Geometry check sheet. Reference: the model listing, model coordinates, mm. A direction names the side the tool comes from. Give positions to 0.01 mm unless a question says otherwise; leave off trailing zeros. Loops run counter-clockwise (first coordinate to the right, second up) from the corner with the lowest first, then second, coordinate; pieces in that order, holes last. Notation, with made-up numbers: (10.25, 52) - (55.25, 52) arc R15 cw to (55.25, 65) - close; hole circle Ø9 at (89, 78.25). An arc over 180 degrees is marked (long way). Use a Markdown table: item, result. Add a question column.
1. Depth check by flat-ended pin: P1, Ø2, axis at x = 217.5, y = -21.5, coming from the +Z side; P2, Ø1.5, axis at x = 241.5, z = -337, coming from the -Y side. Enter the tip coordinate at first touch or a pass-through.
2. Cross-section at B-B on z = -172. Enter the section's corners in (x, y), and give its area (3 significant figures).
3. Material ranges on L1, parallel to Z at x = 308.5, y = -4.5; L2, parallel to X at y = -22.75, z = -360; L3, parallel to Y at x = 265, z = -382.5, recorded low to high.
4. Draft check along Z on faces 3 (the cylindrical face through (7.765, -12.522, -456.036)), 4 (the cylindrical face through (354.185, -12.522, -7.514)), 5 (the flat face through (179, -11, 0)), 6 (the cylindrical face through (356.52, -11.11, -457.82)). Enter one of: pulls with the +Z half, pulls with the -Z half, needs draft (parallel to the pull), parting line crosses it, or undercut.
5. Cross-section at A-A on y = -19.5. Enter the section's corners in (x, z), and give its area (3 significant figures).
6. Set-up check for faces 1 (the cylindrical face through (7.514, -12.522, -7.765)), 2 (the flat face through (0, -11, -235)): record each of +Z, -Z, +X, -X, +Y, -Y from which the full face is reachable in a straight line by a thin tool's end or side.
7. Cross-section at C-C on x = 133. Enter the section's corners in (y, z), and give its area (3 significant figures).
Autodesk Inventor part; units mm, degrees
ref_plane "YZ Plane" through (0, 0, 0) normal (1, 0, 0) x (0, 1, 0)
ref_plane "XZ Plane" through (0, 0, 0) normal (0, 1, 0) x (-1, 0, 0)
ref_plane "XY Plane" through (0, 0, 0) normal (0, 0, 1) x (1, 0, 0)
sketch "Sketch1" plane through (0, 0, 0) normal (0, 1, 0) x (-1, 0, 0)
  line L0 (0, 0) -> (-361.95, 0)
  line L1 (-361.95, 0) -> (-361.95, -463.55)
  line L2 (-361.95, -463.55) -> (0, -463.55)
  line L3 (0, -463.55) -> (0, 0)
  dimension "d0" = 361.95
  dimension "d1" = 463.55
extrude "Extrusion1" add sketch "Sketch1" along normal blind 2.794
fillet "Fillet1" radius 19.05 4 edges at (361.95, 1.397, 0) (361.95, 1.397, -463.55) (0, 1.397, -463.55) (0, 1.397, 0)
sketch "Sketch4" plane through (0, 0, 0) normal (0, -1, 0) x (1, 0, 0)
  point P0 (0, 0)
sketch "Sketch5" plane through (0, 0, 0) normal (0, -1, 0) x (1, 0, 0)
  arc A0 (19.05, 0) -> (0, -19.05) centre (19.05, -19.05) ccw
  line L0 (19.05, 0) -> (342.9, 0)
  line L1 (0, -444.5) -> (0, -19.05)
  line L2 (361.95, -19.05) -> (361.95, -444.5)
  arc A1 (361.95, -19.05) -> (342.9, 0) centre (342.9, -19.05) ccw
  arc A2 (0, -444.5) -> (19.05, -463.55) centre (19.05, -444.5) ccw
  line L3 (342.9, -463.55) -> (19.05, -463.55)
  arc A3 (342.9, -463.55) -> (361.95, -444.5) centre (342.9, -444.5) ccw
  arc A4 (2.9117, -444.5) -> (19.05, -460.6383) centre (19.05, -444.5) ccw
  line L4 (2.9117, -444.5) -> (2.9117, -19.05)
  arc A5 (19.05, -2.9117) -> (2.9117, -19.05) centre (19.05, -19.05) ccw
  line L5 (19.05, -2.9117) -> (342.9, -2.9117)
  arc A6 (359.0383, -19.05) -> (342.9, -2.9117) centre (342.9, -19.05) ccw
  line L6 (359.0383, -19.05) -> (359.0383, -444.5)
  arc A7 (342.9, -460.6383) -> (359.0383, -444.5) centre (342.9, -444.5) ccw
  line L7 (342.9, -460.6383) -> (19.05, -460.6383)
  point P0 (0, 0)
extrude "Extrusion2" add sketch "Sketch5" along normal blind 25.4
properties part number "Cart_LOW_SHELF"
Values found:
| question | item | result |
|---|---|---|
| 1 | P1 | stops at z = 0 |
| 1 | P2 | stops at y = 0 |
| 2 | outline | (0, -25.4) - (2.91, -25.4) - (2.91, 0) - (359.04, 0) - (359.04, -25.4) - (361.95, -25.4) - (361.95, 2.79) - (0, 2.79) - close |
| 2 | area | 1,160 mm2 |
| 3 | L1 | z = -463.55 to -460.64, -2.91 to 0 |
| 3 | L2 | x = 0 to 2.91, 359.04 to 361.95 |
| 3 | L3 | y = 0 to 2.79 |
| 4 | face 3 | undercut |
| 4 | face 4 | undercut |
| 4 | face 5 | pulls with the +Z half |
| 4 | face 6 | pulls with the -Z half |
| 5 | outline | (0, -444.5) arc R19.05 ccw to (19.05, -463.55) - (342.9, -463.55) arc R19.05 ccw to (361.95, -444.5) - (361.95, -19.05) arc R19.05 ccw to (342.9, 0) - (19.05, 0) arc R19.05 ccw to (0, -19.05) - close; hole (2.91, -444.5) arc R16.14 ccw to (19.05, -460.64) - (342.9, -460.64) arc R16.14 ccw to (359.04, -444.5) - (359.04, -19.05) arc R16.14 ccw to (342.9, -2.91) - (19.05, -2.91) arc R16.14 ccw to (2.91, -19.05) - close |
| 5 | area | 4,690 mm2 |
| 6 | face 1 | -Y |
| 6 | face 2 | +Z, -Z, -X, +Y, -Y |
| 7 | outline | (-25.4, -463.55) - (2.79, -463.55) - (2.79, 0) - (-25.4, 0) - (-25.4, -2.91) - (0, -2.91) - (0, -460.64) - (-25.4, -460.64) - close |
| 7 | area | 1,440 mm2 |
